For this review, take the finished solid that the model builds, in its own axes (mm). Face numbers are marked on the shaded views. A direction names the side the tool comes from. Give positions to 0.01 mm unless a question says otherwise; leave off trailing zeros. Order: outer loops, then holes, each group sorted by start corner. A loop starts at its lowest first (then second) coordinate and runs counter-clockwise, first axis right, second up. Notation, with made-up numbers: M -6.5,80 L 51.5,80 A30 cw 51.5,105 Z; hole C 68,14 d9. An arc over 180 degrees is marked long. Answer as CSV lines item,"result". Start each with the question number.
1. For line 1 along X through (y, z) = (27.5, -52.5); line 2 along Y through (x, z) = (65, -24); line 3 along Z through (x, y) = (20.5, 16.5), list the stretches that pass through material, from the lowest coordinate up.
2. We need section D-D, the plane y = 35.5. Give the boundary of the cut face in (x, z), and give its area (3 significant figures).
3. We need section C-C, the plane y = 19.5. Give the boundary of the cut face in (x, z), and give its area (4 significant figures).
4. Mouldability with a two-part tool opening along X and no side actions: class the marked faces 3, 4 and 5 as pulls with the +X half, pulls with the -X half, needs draft (parallel to the pull), parting line crosses it, or undercut.
5. We need section B-B, the plane z = -85. Give the boundary of the cut face in (x, y).
6. Machinability: for the marked faces 1 and 2, which of the approach directions +Z, -Z, +X, -X, +Y, -Y give a long, thin tool a straight path to every point of the face, cutting with its end or side? Answer none if there is none.
7. Clearance check with flat-ended pins moving along their axes: P1, Ø16.5, axis at x = 63.5, y = 18, coming from the -Z side; P2, Ø6, axis at y = 31.5, z = -37.5, coming from the -X side; P3, Ø1.5, axis at y = 5, z = -66, coming from the +X side. State where each tip first meets the part, or that it passes through.
8. We need section A-A, the plane x = 4. Give the boundary of the cut face in (y, z), and give its area (3 significant figures).
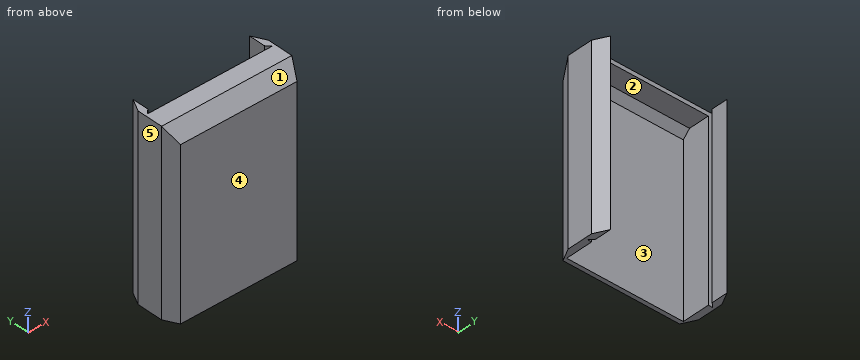
from build123d import *

# Parameters (mm, degrees)
SKETCH1_W                           = 85
SKETCH1_H                           = 130
BOSS_EXTRUDE1_BASE_DEPTH            = 3
BOSS_EXTRUDE4_SIDE_WALLS_DEPTH      = 130
CUT_EXTRUDE2_GUIDE_HOLES_DEPTH      = 163.616112363
SKETCH15_W                          = 85
SKETCH15_H                          = 20
BOSS_EXTRUDE9_FRONT_WALL_DEPTH      = 3
CHAMFER5_FRONT_CHAMFER_SIZE         = 9.61
CHAMFER6_FRONT_CHAMFER_CLEANUP_SIZE = 5


with BuildPart() as part:
    # Sketch1 → Boss-Extrude1 (Base) (new body)
    with BuildSketch(Plane(origin=(0, 0, 0), x_dir=(1, 0, 0), z_dir=(0, 1, 0))):
        with Locations((42.5, 65)):
            Rectangle(SKETCH1_W, SKETCH1_H)
    extrude(amount=BOSS_EXTRUDE1_BASE_DEPTH)

    # Sketch5 → Boss-Extrude4 (Side Walls) (add, through all)
    with BuildSketch(Plane.XY):
        Polygon((-5, 28.390936655), (0, 38), (0, 0), (-5, 9.609063345), align=None)
        Polygon((90, 9.609063345), (90, 28.390936655), (85, 38), (85, 0), align=None)
    extrude(amount=-BOSS_EXTRUDE4_SIDE_WALLS_DEPTH)

    # Sketch4 → Cut-Extrude2 (Guide Holes) (cut, through all)
    with BuildSketch(Plane.XY):
        Polygon((-3.1, 23), (0, 26.1), (0, 23), align=None)
        Polygon((85, 23), (88.1, 23), (85, 26.1), align=None)
    extrude(amount=-CUT_EXTRUDE2_GUIDE_HOLES_DEPTH, mode=Mode.SUBTRACT)

    # Sketch15 → Boss-Extrude9 (Front Wall) (add)
    with BuildSketch(Plane.XY):
        with Locations((42.5, 13)):
            Rectangle(SKETCH15_W, SKETCH15_H)
    extrude(amount=-BOSS_EXTRUDE9_FRONT_WALL_DEPTH)

    # Chamfer5 (Front Chamfer)
    chamfer5_front_chamfer_edges = [part.edges().sort_by_distance(p)[0] for p in [
        (42.5, 0, 0),
    ]]
    chamfer(chamfer5_front_chamfer_edges, length=CHAMFER5_FRONT_CHAMFER_SIZE)

    # Chamfer6 (Front Chamfer Cleanup)
    chamfer6_front_chamfer_cleanup_edges = [part.edges().sort_by_distance(p)[0] for p in [
        (42.5, 3, -3),
    ]]
    chamfer(chamfer6_front_chamfer_cleanup_edges, length=CHAMFER6_FRONT_CHAMFER_CLEANUP_SIZE)


solid = part.part
Result set:
1,line 1,"-5 to 0, 85 to 90"
1,line 2,"0 to 3"
1,line 3,"-3 to 0"
2,outline,"M -1.3,-130 L 0,-130 L 0,0 L -1.3,0 Z; M 85,-130 L 86.3,-130 L 86.3,0 L 85,0 Z"
2,area,"338 mm2"
3,outline,"M -5,-130 L 0,-130 L 0,-3 L 85,-3 L 85,-130 L 90,-130 L 90,0 L -5,0 Z"
3,area,"1,555 mm2"
4,face 3,"undercut"
4,face 4,"needs draft"
4,face 5,"pulls with the -X half"
5,outline,"M -5,9.61 L 0,0 L 85,0 L 90,9.61 L 90,28.39 L 85,38 L 85,26.1 L 88.1,23 L 85,23 L 85,3 L 0,3 L 0,23 L -3.1,23 L 0,26.1 L 0,38 L -5,28.39 Z"
6,face 1,"+Z, +X, -X, -Y"
6,face 2,"-Z, +Y"
7,P1,"z = -3"
7,P2,"x = -4.94"
7,P3,"x = 87.99"
8,outline,"M 0,-130 L 3,-130 L 3,-8 L 8,-3 L 23,-3 L 23,0 L 9.61,0 L 0,-9.61 Z"
8,area,"416 mm2"
